Here's how the part is built. I have some questions about the finished solid (model axes, mm). A direction names the side the tool comes from. Give positions to 0.01 mm unless a question says otherwise; leave off trailing zeros. Write each loop counter-clockwise with the first axis right and the second up, starting at its lowest first coordinate (ties: lowest second). Pieces come first, ordered by that corner, then holes. Notation, with made-up numbers: (22, 84.5) - (58, 84.5) arc R21 ccw to (58, 111.5) - close; hole circle Ø5 at (70, 25). An arc over 180 degrees is marked (long way). One line per item, written item: value. Start each with the question number.
1) On a 3-axis mill with a long thin cutter (end or side, diameter ignored), from which of +Z, -Z, +X, -X, +Y, -Y can I reach the whole of each face in a straight line? I mean faces 1 (the cylindrical face through (5.17, 236.48, -0.99)), 2 (the flat face through (2, 125, -21)). Say none if no direction works.
2) Imagine slicing it at D-D on y = 28. Write out the boundary of the cut face in (x, z), plus the area to 3 significant figures.
3) Imagine slicing it at A-A on x = 5.5. Write out the boundary of the cut face in (y, z), plus the area to 3 significant figures.
4) Imagine slicing it at C-C on z = -30. Write out the boundary of the cut face in (x, y), plus the area to 3 significant figures.
5) Imagine slicing it at B-B on y = 234. Write out the boundary of the cut face in (x, z), plus the area to 3 significant figures.
6) Please list where these lines run through material, in increasing order: L1, parallel to Y at x = 5.5, z = -39.6; L2, parallel to X at y = 234, z = -0.65; L3, parallel to Z at x = 10.25, y = 72. Write a range as [from, to].
7) I'm going to push flat-ended pins straight in: P1, Ø5, axis at x = 5.5, z = -9.5, coming from the -Y side; P2, Ø6, axis at x = 5.5, y = 234, coming from the -Z side. Where does each tip first touch, or does it pass through?
8) We'd pull the mould along Y, two halves only. Please class faces 3 (the flat face through (1, 254, -16)), 4 (the flat face through (6, 125, 0)), 5 (the cylindrical face through (5.17, 236.48, -39.99)): +Y half, -Y half, draft (parallel to the pull), parting line (faces both ways), or undercut.
from build123d import *

# Parameters (mm, degrees)
BOSS_EXTRUDE1_DEPTH = 254
SKETCH2_R           = 2.5
CUT_EXTRUDE1_DEPTH  = 42


with BuildPart() as part:
    # Sketch1 → Boss-Extrude1 (new body)
    with BuildSketch(Plane(origin=(0, 0, 0), x_dir=(1, 0, 0), z_dir=(0, 1, 0))):
        Polygon((0, 0), (0, 41), (11, 41), (11, 39), (2, 39), (2, 2), (11, 2), (11, 0), align=None)
    extrude(amount=BOSS_EXTRUDE1_DEPTH)

    # Sketch2 → Cut-Extrude1 (cut, through all)
    with BuildSketch(Plane.XY):
        with Locations((5.5, 234)):
            Circle(SKETCH2_R)
    extrude(amount=-CUT_EXTRUDE1_DEPTH, mode=Mode.SUBTRACT)


solid = part.part
Numbers:
1. face 1: +Z, -Z
1. face 2: +X, +Y, -Y
2. outline: (0, -41) - (11, -41) - (11, -39) - (2, -39) - (2, -2) - (11, -2) - (11, 0) - (0, 0) - close
2. area: 118 mm^2
3. outline: (0, -41) - (231.5, -41) - (231.5, -39) - (0, -39) - close; (0, -2) - (231.5, -2) - (231.5, 0) - (0, 0) - close; (236.5, -41) - (254, -41) - (254, -39) - (236.5, -39) - close; (236.5, -2) - (254, -2) - (254, 0) - (236.5, 0) - close
3. area: 996 mm^2
4. outline: (0, 0) - (2, 0) - (2, 254) - (0, 254) - close
4. area: 508 mm^2
5. outline: (0, -41) - (3, -41) - (3, -39) - (2, -39) - (2, -2) - (3, -2) - (3, 0) - (0, 0) - close; (8, -41) - (11, -41) - (11, -39) - (8, -39) - close; (8, -2) - (11, -2) - (11, 0) - (8, 0) - close
5. area: 98.0 mm^2
6. L1: [0, 231.5], [236.5, 254]
6. L2: [0, 3], [8, 11]
6. L3: [-41, -39], [-2, 0]
7. P1: through
7. P2: z = -41
8. face 3: +Y half
8. face 4: draft
8. face 5: undercut
